from build123d import *

# Parameters (mm, degrees)
F0_R           = 12.7
F1_DEPTH       = 76.2
F3_R           = 6.35
F4_DEPTH       = 19.05
F5_R           = 6.35
F6_DEPTH       = 11.938
F7_DEPTH       = 19.05
F8_R           = 5.08
F9_R           = 1.27
F10_DEPTH      = 25.4
F10_DEPTH_BACK = 25.4


with BuildPart() as f1:
    # F0 (on Front) → F1 (new body)
    with BuildSketch(Plane.XZ):
        Circle(F0_R)
    extrude(amount=-F1_DEPTH)

    # F3 (on face) → F4 (cut)
    with BuildSketch(Plane.XZ):
        Circle(F3_R)
    extrude(amount=-F4_DEPTH, mode=Mode.SUBTRACT)

    # F5 (on face) → F6 (join)
    with BuildSketch(Plane.XZ):
        Circle(F5_R)
    extrude(amount=-F6_DEPTH)

    # F2 (on face) → F7 (cut)
    with BuildSketch(Plane.XZ):
        Polygon((5.08, -2.54), (5.08, 0), (5.08, 2.54), (-5.08, 2.54), (-5.08, -2.54), align=None)
    extrude(amount=-F7_DEPTH, mode=Mode.SUBTRACT)

    # F8
    f8_edges = [f1.edges().sort_by_distance(p)[0] for p in [
        (-12.7, 76.2, 0),
    ]]
    fillet(f8_edges, radius=F8_R)

    # F9 (on Top) → F10 (cut, two sides)
    with BuildSketch(Plane.XY) as f10_sk:
        with Locations((9.823189, 2.76481)):
            Circle(F9_R)
    extrude(amount=F10_DEPTH, mode=Mode.SUBTRACT)
    extrude(f10_sk.sketch, amount=-F10_DEPTH_BACK, mode=Mode.SUBTRACT)


solid = f1.part
CAD build for the part. Positions are in the model's coordinates, mm. A direction names the side the tool comes from. Round coordinates to 2 decimals unless told otherwise and drop trailing zeros. Order: outer loops, then holes, each group sorted by start corner. A loop starts at its lowest first (then second) coordinate and runs counter-clockwise, first axis right, second up. Notation, with made-up numbers: (26, 62) -> (60, 62) arc R11 ccw to (60, 80) -> close; hole circle Ø9 at (62.5, 51). An arc over 180 degrees is marked (long way). Write each question's results on one line, items separated by ' | '.
1. Cut at B-B (y = 7). Give the cut face in (x, z), plus the area to 3 significant figures.
Findings below:
outline: circle Ø25.4 at (0, 0); hole (-5.08, -2.54) -> (5.08, -2.54) -> (5.08, 2.54) -> (-5.08, 2.54) -> close | area: 455 mm²
2. Cut at C-C (y = 20.5). Give the cut face in (x, z), plus the area to 3 significant figures.
Findings below:
outline: circle Ø25.4 at (0, 0) | area: 507 mm²
3. Cut at D-D (z = 5.5). Count the separate pieces of the cut face and the enclosed holes in it, plus the area to 3 significant figures.
Findings below:
separate pieces: 1 | enclosed holes: 2 | area: 1,680 mm²
4. Cut at A-A (x = 0). Give the cut face in (y, z), plus the area to 3 significant figures.
Findings below:
outline: (0, -12.7) -> (71.12, -12.7) arc R5.08 ccw to (76.2, -7.62) -> (76.2, 7.62) arc R5.08 ccw to (71.12, 12.7) -> (0, 12.7) -> (0, 2.54) -> (11.94, 2.54) -> (11.94, 6.35) -> (19.05, 6.35) -> (19.05, -6.35) -> (11.94, -6.35) -> (11.94, -2.54) -> (0, -2.54) -> close | area: 1,770 mm²
5. Flat gauge pins, fed straight in: P1, Ø4, axis at x = 3, z = 3, coming from the -Y side; P2, Ø1.5, axis at y = 6.5, z = -1, coming from the +X side; P3, Ø2, axis at x = -2.5, y = 8.5, coming from the -Z side; P4, Ø3, axis at x = 9.82, y = 2.76, coming from the +Z side. Where does each tip first touch, or does it go through?
Findings below:
P1: stops at y = 0 | P2: stops at x = 12.7 | P3: stops at z = -12.61 | P4: stops at z = 9.6
6. Pull direction Y, two halves, no side cores. Call faces 4 (the face through (0, 0, -3)), 5 (the face through (0, 11.938, -3)), 6 (the face through (-5.08, 6, 0)): pulls with the +Y half, pulls with the -Y half, needs draft (parallel to the pull), parting line crosses it, or undercut.
Findings below:
face 4: pulls with the -Y half | face 5: undercut | face 6: needs draft
7. 3-axis set-ups, long thin cutter, end or side, ignore diameter. For faces 1 (the face through (-2.75, 35.06, -12.4)), 2 (the face through (0, 6, -2.54)), 3 (the face through (0, 19.05, 0)): which of +Z, -Z, +X, -X, +Y, -Y reach the whole face in a straight line?
Findings below:
face 1: +Y, -Y | face 2: -Y | face 3: none
8. Wall check: line 1 along Y through (x, z) = (-2, -5.5); line 2 along Z through (x, y) = (0, 16); line 3 along Z through (x, y) = (-4.5, 9.5). Give the ranges that are in metal, low to high. Write a range as [from, to].
Findings below:
line 1: y = [0, 11.94], [19.05, 76.2] | line 2: z = [-12.7, -6.35], [6.35, 12.7] | line 3: z = [-11.88, -2.54], [2.54, 11.88]
